Geometry check sheet. Reference: the model listing, model coordinates, mm. Face numbers are marked on the shaded views. A direction names the side the tool comes from. Round coordinates to 2 decimals unless told otherwise and drop trailing zeros. Write each loop counter-clockwise with the first axis right and the second up, starting at its lowest first coordinate (ties: lowest second). Pieces come first, ordered by that corner, then holes. Notation, with made-up numbers: (85, 15) -> (118, 15) arc R29 cw to (118, 43) -> close; hole circle Ø3 at (42.5, 37). An arc over 180 degrees is marked (long way). Return JSON: item names as keys, results as strings. Group by question number.
Autodesk Inventor part; units mm, degrees
ref_plane "YZ Plane" through (0, 0, 0) normal (1, 0, 0) x (0, 1, 0)
ref_plane "XZ Plane" through (0, 0, 0) normal (0, 1, 0) x (-1, 0, 0)
ref_plane "XY Plane" through (0, 0, 0) normal (0, 0, 1) x (1, 0, 0)
sketch "Sketch1" plane through (0, 0, 0) normal (0, 0, 1) x (1, 0, 0)
  circle A0 centre (0, 0) radius 9.525
  line L0 (0, -7.3323) -> (-6.35, -3.6662)
  line L1 (-6.35, -3.6662) -> (-6.35, 3.6662)
  line L2 (-6.35, 3.6662) -> (0, 7.3323)
  line L3 (0, 7.3323) -> (6.35, 3.6662)
  line L4 (6.35, 3.6662) -> (6.35, -3.6662)
  line L5 (6.35, -3.6662) -> (0, -7.3323)
  dimension "d0" = 19.05
  dimension "d1" = 12.7
extrude "Extrusion1" add sketch "Sketch1" along normal mid plane 12.7
properties part number "500 Hex Spacer 0.5"
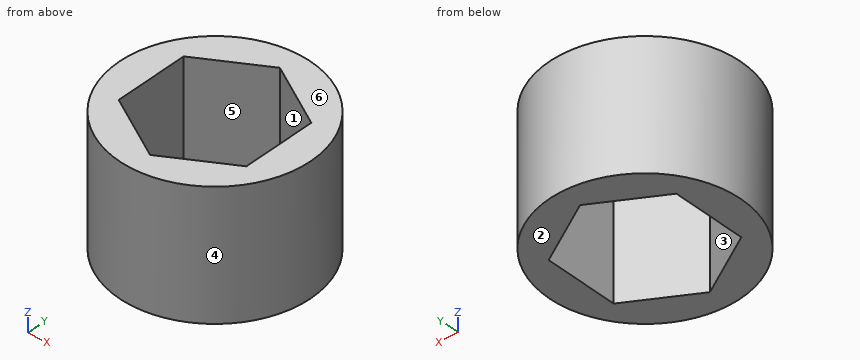
1) Tool access check on the marked faces 5 and 6. Record the directions out of +Z, -Z, +X, -X, +Y, -Y that give a thin tool (end or side, any length) a straight path to the whole face; none if there is none.
2) Sectioned sample at B-B on y = 0. Enter the section's corners in (x, z) (3 decimals), and give its area (3 significant figures).
3) Mould release check, pull along X, two halves, no side actions. Record for the marked faces 1, 2, 3 and 4: +X half, -X half, draft (parallel to the pull), parting line (faces both ways), or undercut.
4) Material ranges on probe 1 along X at (y, z) = (3.5, 5); probe 2 along Y at (x, z) = (-5.75, 5.25); probe 3 along X at (y, z) = (7.25, 1), recorded low to high. Write a range as [from, to].
5) Sectioned sample at A-A on z = -3.5. Enter the section's corners in (x, y) (3 decimals), and give its area (3 significant figures).
6) Sectioned sample at D-D on y = 8.75. Enter the section's corners in (x, z), and give its area (3 significant figures).
7) Go/stop test with flat-tipped pins: P1, Ø1.5, axis at x = -6, z = 0, coming from the +Y side; P2, Ø3, axis at x = 6.5, z = -3.5, coming from the +Y side; P3, Ø2, axis at y = 1.5, z = -2.5, coming from the +X side. Record where each tip stops, or that it passes through.
8) Sectioned sample at C-C on x = -2.5. Enter the section's corners in (y, z), and give its area (3 significant figures).
Evaluation:
{
 "1": {"face 5": "+Z, -Z", "face 6": "+Z, +X, -X, +Y, -Y"},
 "2": {"outline": "(-9.525, -6.35) -> (-6.35, -6.35) -> (-6.35, 6.35) -> (-9.525, 6.35) -> close; (6.35, -6.35) -> (9.525, -6.35) -> (9.525, 6.35) -> (6.35, 6.35) -> close", "area": "80.6 mm2"},
 "3": {"face 1": "undercut", "face 2": "draft", "face 3": "undercut", "face 4": "parting line"},
 "4": {"probe 1": "x = [-8.86, -6.35], [6.35, 8.86]", "probe 2": "y = [-7.59, -4.01], [4.01, 7.59]", "probe 3": "x = [-6.18, -0.14], [0.14, 6.18]"},
 "5": {"outline": "circle Ø19.05 at (0, 0); hole (-6.35, -3.666) -> (0, -7.332) -> (6.35, -3.666) -> (6.35, 3.666) -> (0, 7.332) -> (-6.35, 3.666) -> close", "area": "145 mm2"},
 "6": {"outline": "(-3.76, -6.35) -> (3.76, -6.35) -> (3.76, 6.35) -> (-3.76, 6.35) -> close", "area": "95.6 mm2"},
 "7": {"P1": "stops at y = 7.95", "P2": "stops at y = 8.11", "P3": "stops at x = 9.51"},
 "8": {"outline": "(-9.19, -6.35) -> (-5.89, -6.35) -> (-5.89, 6.35) -> (-9.19, 6.35) -> close; (5.89, -6.35) -> (9.19, -6.35) -> (9.19, 6.35) -> (5.89, 6.35) -> close", "area": "83.9 mm2"}
}
